from build123d import *

# Parameters (mm, degrees)
BOSS_EXTRU_1_DEPTH      = 20
CONG_1_R                = 5
CHANFREIN1_SIZE2        = 5
CHANFREIN1_SIZE         = 3.535545122
BOSS_EXTRU_2_DEPTH      = 4
ESQUISSE9_W             = 20
ESQUISSE9_H             = 48.160254038
ENL_V_MAT_EXTRU_5_DEPTH = 2
ESQUISSE10_R            = 6.5
ENL_V_MAT_EXTRU_6_DEPTH = 4


with BuildPart() as part:
    # Esquisse1 → Boss.-Extru.1 (new body)
    with BuildSketch(Plane.XY.offset(164.870489571)):
        Polygon((-68.588600326, 5.142765071), (-68.588600326, 15.502551901), (-78.588600326, 12.796044343), (-90.211700696, 9.650243444), (-68.996801706, 46.395526372), (-72.460903321, 48.395526372), (-102.774849854, -4.109769201), (-78.588600326, 2.436257514), (-78.588600326, -32.657702137), (-68.588600326, -32.657702137), align=None)
    extrude(amount=-BOSS_EXTRU_1_DEPTH)

    # Congé1
    cong_1_edges = [part.edges().sort_by_distance(p)[0] for p in [
        (-90.211700696, 9.650243444, 154.870489571),
        (-78.588600326, 2.436257514, 154.870489571),
    ]]
    fillet(cong_1_edges, radius=CONG_1_R)

    # Chanfrein1
    chanfrein1_edges = [part.edges().sort_by_distance(p)[0] for p in [
        (-102.774849854, -4.109769201, 154.870489571),
    ]]
    chamfer(chanfrein1_edges, length=CHANFREIN1_SIZE, length2=CHANFREIN1_SIZE2)

    # Esquisse8 → Boss.-Extru.2 (add)
    with BuildSketch(Plane(origin=(-75.301555125, 43.475373122, 0), x_dir=(0, 0, 1), z_dir=(-0.866025404, 0.5, 0))):
        with BuildLine():
            Line((144.870489571, 5.681303607), (164.870489571, 5.681303607))
            ThreePointArc((164.870489571, 5.681303607), (154.870489571, 15.681303607), (144.870489571, 5.681303607))
        make_face()
    extrude(amount=-BOSS_EXTRU_2_DEPTH)

    # Esquisse9 → Enlèv. mat.-Extru.5 (cut)
    with BuildSketch(Plane(origin=(-68.588600326, 0, 0), x_dir=(0, 0, -1), z_dir=(1, 0, 0))):
        with Locations((-154.870489571, -8.577575118)):
            Rectangle(ESQUISSE9_W, ESQUISSE9_H)
    extrude(amount=-ENL_V_MAT_EXTRU_5_DEPTH, mode=Mode.SUBTRACT)

    # Esquisse10 → Enlèv. mat.-Extru.6 (cut)
    with BuildSketch(Plane(origin=(-75.301555125, 43.475373122, 0), x_dir=(0, 0, 1), z_dir=(-0.866025404, 0.5, 0))):
        with Locations((154.870489571, -11.868696393)):
            Circle(ESQUISSE10_R)
    extrude(amount=-ENL_V_MAT_EXTRU_6_DEPTH, mode=Mode.SUBTRACT)


solid = part.part
The listing builds one solid part. Answer for the finished solid, in the listing's coordinates (mm). A direction names the side the tool comes from. Give positions to 0.01 mm unless a question says otherwise; leave off trailing zeros. Write each loop counter-clockwise with the first axis right and the second up, starting at its lowest first coordinate (ties: lowest second). Pieces come first, ordered by that corner, then holes.
1) Section A-A (y = 22.5) is taken. Write down the section's boundary in (x, z), and give its area (3 significant figures).
2) A tool of negligible diameter and unlimited length cuts with its end or side. For faces 4 (the face through (-65.754, 56.068, 155.09)), 5 (the face through (-74.498, 13.903, 155.01)), 6 (the face through (-70.589, -9, 155)), 7 (the face through (-78.589, -18, 155)), from which of +Z, -Z, +X, -X, +Y, -Y can it reach the whole face along a straight path? Write none if from no direction.
3) Section B-B (x = -90.5) is taken. Write down the section's boundary in (y, z), and give its area (3 significant figures).
4) Find the intervals of material crossed by L1, parallel to X at y = -21.5, z = 155.75; L2, parallel to Y at x = -80.5, z = 160.5; L3, parallel to Y at x = -84, z = 146.25, in increasing order.
5) For a pull along Z with two mould halves and no side action, classify faces 1 (the face through (-83, 5, 144.87)), 2 (the face through (-79.385, 32.458, 148.377)), 3 (the face through (-91.51, -1.06, 155.01)) as pulls with the +Z half, pulls with the -Z half, needs draft (parallel to the pull), parting line crosses it, or undercut.
6) Given P1, Ø8, axis at y = -20.5, z = 156, coming from the +X side; P2, Ø1.5, axis at y = 28.5, z = 157.5, coming from the -X side; P3, Ø3, axis at x = -89, y = 21.5, coming from the +Z side; P4, Ø4, axis at x = -78.5, z = 161, coming from the +Y side, each flat-ended and moving along its own axis, determine where each tip first touches the part or whether it passes through.
Response:
1. outline: (-87.41, 144.87) - (-82.79, 144.87) - (-82.79, 164.87) - (-87.41, 164.87) - close
1. area: 92.4 mm2
2. face 4: +X, +Y
2. face 5: +Z, -Z
2. face 6: +Z, -Z, +X, -Y
2. face 7: +Z, -Z, -X, -Y
3. outline: (-0.79, 144.87) - (17.15, 144.87) - (17.15, 164.87) - (-0.79, 164.87) - close
3. area: 359 mm2
4. L1: x = -78.59 to -70.59
4. L2: y = -0.16 to 12.69, 26.47 to 29.02
4. L3: y = 0.89 to 14.89, 20.41 to 28.41
5. face 1: pulls with the -Z half
5. face 2: undercut
5. face 3: needs draft
6. P1: stops at x = -70.59
6. P2: stops at x = -84.38
6. P3: stops at z = 164.87
6. P4: stops at y = 41.4
